Input: part model. Units: mm. Frame: model coordinates. Round coordinates to 2 decimals unless told otherwise and drop trailing zeros. Order: outer loops, then holes, each group sorted by start corner. A loop starts at its lowest first (then second) coordinate and runs counter-clockwise, first axis right, second up. Notation, with made-up numbers: (32, -40) -> (78, -40) arc R15 ccw to (78, -35) -> close; hole circle Ø8 at (-40, -39). An arc over 180 degrees is marked (long way). Use a Markdown table: item, result.
from build123d import *

# Parameters (mm, degrees)
SKETCH1_R         = 2
EXTRUDE1_DEPTH    = 78
SKETCH2_R         = 3.35
EXTRUDE2_DEPTH    = 1
DOME1_FACE_RADIUS = 3.35
DOME1_HEIGHT      = 2


with BuildPart() as part:
    # Sketch1 → Extrude1 (new body)
    with BuildSketch(Plane.XY):
        Circle(SKETCH1_R)
    extrude(amount=EXTRUDE1_DEPTH)

    # Sketch2 → Extrude2 (add)
    with BuildSketch(Plane(origin=(0, 0, 0), x_dir=(-1, 0, 0), z_dir=(0, 0, -1))):
        Circle(SKETCH2_R)
    extrude(amount=EXTRUDE2_DEPTH)

    # Dome1: a dome of height H over a round flat face of radius A is a cap of a sphere of radius (A * A + H * H) / (2 * H)
    dome1_r = (DOME1_FACE_RADIUS * DOME1_FACE_RADIUS + DOME1_HEIGHT * DOME1_HEIGHT) / (2 * DOME1_HEIGHT)
    dome1_base = Plane((0, 0, -1), z_dir=(0, 0, -1))
    with Locations(dome1_base.offset(DOME1_HEIGHT - dome1_r)):
        dome1_ball = Sphere(dome1_r, mode=Mode.PRIVATE)
    add(split(dome1_ball, bisect_by=dome1_base, keep=Keep.TOP, mode=Mode.PRIVATE))


solid = part.part
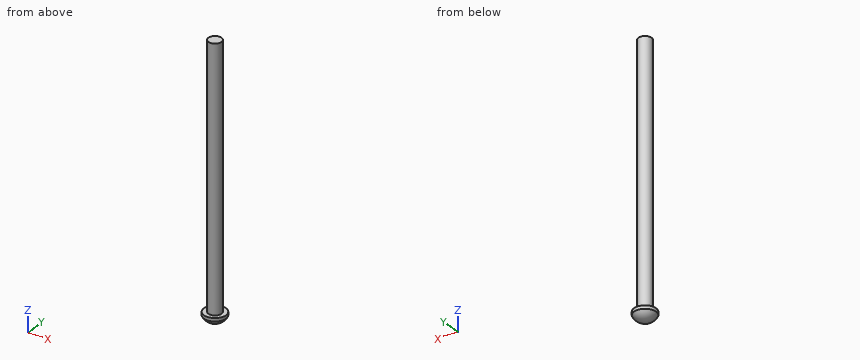
1) Cut plane C-C on z = 55.5. Return loops of the section in (x, y), and give its area (3 significant figures).
Results found:
| item | result |
|---|---|
| outline | circle Ø4 at (0, 0) |
| area | 12.6 mm² |
2) Cut plane A-A on x = 0. Return loops of the section in (y, z).
Results found:
| item | result |
|---|---|
| outline | (-3.35, -1) arc R3.81 ccw to (3.35, -1) -> (3.35, 0) -> (2, 0) -> (2, 78) -> (-2, 78) -> (-2, 0) -> (-3.35, 0) -> close |
3) Pin query (flat end, axial travel): pin 1 Ø1.5 at (x, z) = (-1, 36) entering from -Y; pin 2 Ø1 at (x, y) = (1.5, 0) entering from -Z; pin 3 Ø3 at (x, y) = (-2.5, 0) entering from +Z. Return the tip coordinate at first contact, or that it passes through.
Results found:
| item | result |
|---|---|
| pin 1 | stops at y = -1.98 |
| pin 2 | stops at z = -2.87 |
| pin 3 | stops at z = 78 |
4) Line query: L1, parallel to X at y = -0.25, z = 34; L2, parallel to X at y = -1.5, z = 52.5. Output: solid intervals per line, ascending. Write a range as [from, to].
Results found:
| item | result |
|---|---|
| L1 | x = [-1.98, 1.98] |
| L2 | x = [-1.32, 1.32] |
